Check sheet for the drawn part. Datum: minimum x, y, z corner. Units: mm. A direction names the side the tool comes from. Round coordinates to 2 decimals unless told otherwise and drop trailing zeros. Order: outer loops, then holes, each group sorted by start corner. A loop starts at its lowest first (then second) coordinate and runs counter-clockwise, first axis right, second up. Notation, with made-up numbers: (-17.75, 48.25) -> (17.25, 48.25) arc R31 cw to (17.25, 74.25) -> close; hole circle Ø1 at (54.5, 78.5). An arc over 180 degrees is marked (long way). Answer as CSV lines item,"result". Start each with the question number.
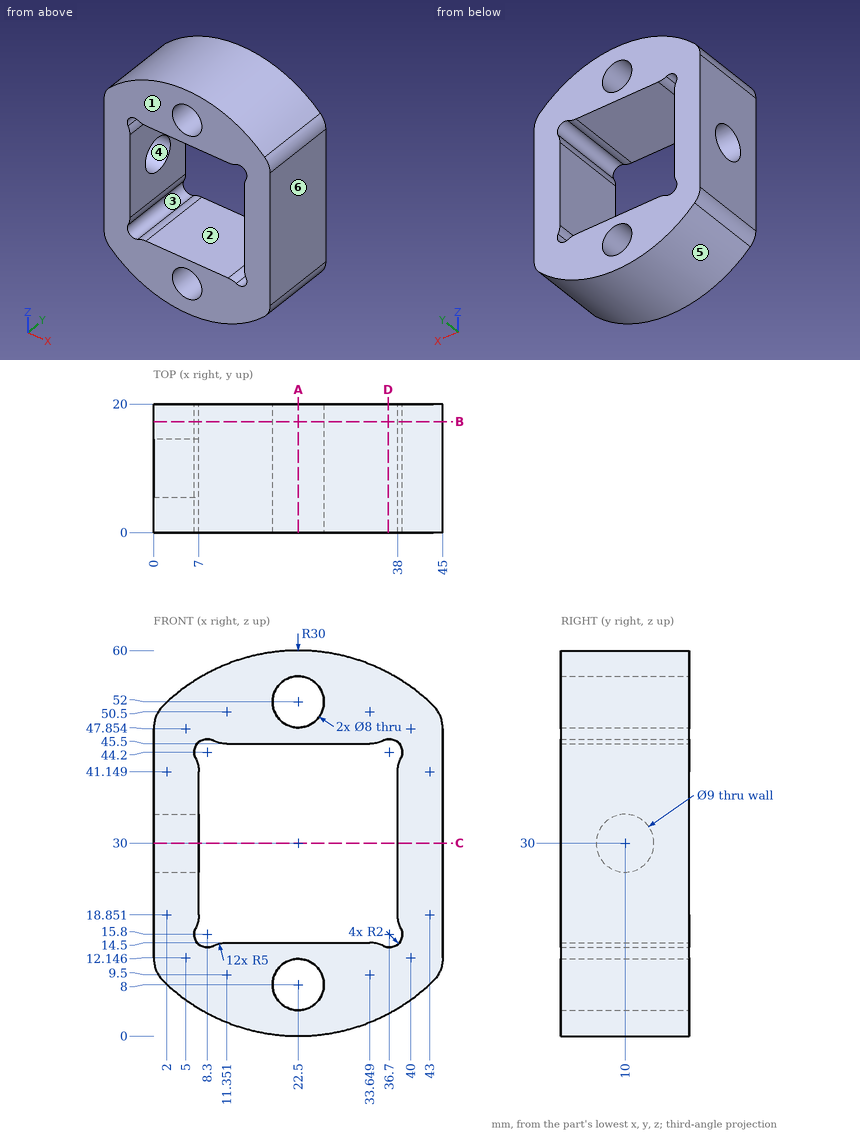
1) Section check A-A on x = 22.5. Record the cut outline in (y, z).
2) Access from +Z, -Z, +X, -X, +Y, -Y to the whole of each face (thin tool, end or side, straight path). Record for the marked faces 1 and 2.
3) Section check B-B on y = 17.25. Record the cut outline in (x, z) (1 decimal), then the cut area to 3 significant figures.
4) Mould release check, pull along Z, two halves, no side actions. Record for the marked faces 3, 4, 5 and 6: released by +Z, released by -Z, zero draft, split by the parting line, or undercut.
5) Section check C-C on z = 30. Record the cut outline in (x, y), then the cut area to 3 significant figures.
6) Depth check by flat-ended pin: pin 1 Ø8 at (x, y) = (7, 4.5) entering from +Z; pin 2 Ø2 at (x, y) = (37, 13.5) entering from +Z. Enter the tip coordinate at first touch or a pass-through.
7) Material ranges on line 1 along X through (y, z) = (3, 28.5); line 2 along Z through (x, y) = (32, 6.5) (1 decimal); line 3 along Z through (x, y) = (4.5, 10), recorded low to high.
8) Section check D-D on x = 36.5. Record the cut outline in (y, z), then the cut area to 3 significant figures.
Solutions:
1,outline,"(0, 0) -> (20, 0) -> (20, 4) -> (0, 4) -> close; (0, 12) -> (20, 12) -> (20, 14.5) -> (0, 14.5) -> close; (0, 45.5) -> (20, 45.5) -> (20, 48) -> (0, 48) -> close; (0, 56) -> (20, 56) -> (20, 60) -> (0, 60) -> close"
2,face 1,"+Z, -Z, +X, -X, -Y"
2,face 2,"+Y, -Y"
3,outline,"(0, 12.1) arc R5 ccw to (1.5, 8.6) arc R30 ccw to (43.5, 8.6) arc R5 ccw to (45, 12.1) -> (45, 47.9) arc R5 ccw to (43.5, 51.4) arc R30 ccw to (1.5, 51.4) arc R5 ccw to (0, 47.9) -> close; hole (6.5, 16.7) arc R2 ccw to (9.2, 14) arc R5 cw to (11.4, 14.5) -> (33.6, 14.5) arc R5 cw to (35.8, 14) arc R2 ccw to (38.5, 16.7) arc R5 cw to (38, 18.9) -> (38, 41.1) arc R5 cw to (38.5, 43.3) arc R2 ccw to (35.8, 46) arc R5 cw to (33.6, 45.5) -> (11.4, 45.5) arc R5 cw to (9.2, 46) arc R2 ccw to (6.5, 43.3) arc R5 cw to (7, 41.1) -> (7, 18.9) arc R5 cw to start; hole circle Ø8 at (22.5, 8); hole circle Ø8 at (22.5, 52)"
3,area,"1,340 mm^2"
4,face 3,"undercut"
4,face 4,"undercut"
4,face 5,"released by -Z"
4,face 6,"zero draft"
5,outline,"(0, 0) -> (7, 0) -> (7, 5.5) -> (0, 5.5) -> close; (0, 14.5) -> (7, 14.5) -> (7, 20) -> (0, 20) -> close; (38, 0) -> (45, 0) -> (45, 20) -> (38, 20) -> close"
5,area,"217 mm^2"
6,pin 1,"stops at z = 57.71"
6,pin 2,"stops at z = 56.79"
7,line 1,"x = 0 to 7, 38 to 45"
7,line 2,"z = 1.5 to 14.5, 45.5 to 58.5"
7,line 3,"z = 6 to 25.5, 34.5 to 54"
8,outline,"(0, 3.47) -> (20, 3.47) -> (20, 13.81) -> (0, 13.81) -> close; (0, 46.19) -> (20, 46.19) -> (20, 56.53) -> (0, 56.53) -> close"
8,area,"414 mm^2"
